The listing builds one solid part. Answer for the finished solid, in the listing's coordinates (mm). Face numbers are marked on the shaded views. A direction names the side the tool comes from. Coordinates: 2 decimals unless noted, no trailing zeros. Order: outer loops, then holes, each group sorted by start corner. A loop starts at its lowest first (then second) coordinate and runs counter-clockwise, first axis right, second up.
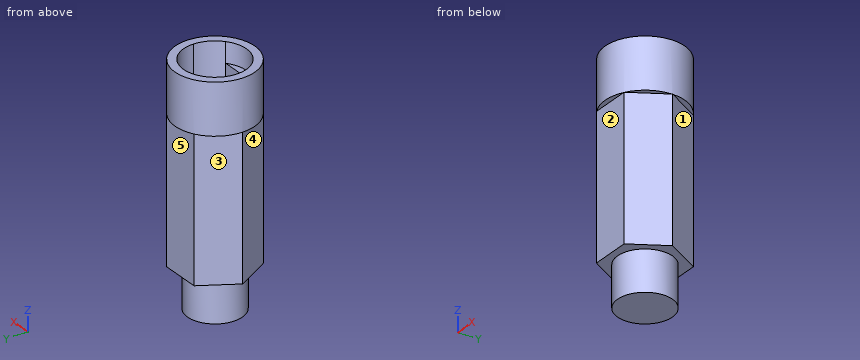
```python
from build123d import *

# Parameters (mm, degrees)
BOSS_EXTRUDE1_DEPTH = 14
SKETCH2_R           = 3.925
BOSS_EXTRUDE2_DEPTH = 5
SKETCH3_R           = 2.7
BOSS_EXTRUDE3_DEPTH = 4
CUT_EXTRUDE1_DEPTH  = 16
SKETCH5_R           = 3.1
CUT_EXTRUDE2_DEPTH  = 2


with BuildPart() as part:
    # Sketch1 → Boss-Extrude1 (new body)
    with BuildSketch(Plane.XY):
        Polygon((3.95, 0), (1.975, 3.420800345), (-1.975, 3.420800345), (-3.95, 0), (-1.975, -3.420800345), (1.975, -3.420800345), align=None)
    extrude(amount=BOSS_EXTRUDE1_DEPTH)

    # Sketch2 → Boss-Extrude2 (add)
    with BuildSketch(Plane.XY.offset(14)):
        with Locations(Location((0, 0, 0), (0, 0, 180.63826759))):
            Circle(SKETCH2_R)
    extrude(amount=BOSS_EXTRUDE2_DEPTH)

    # Sketch3 → Boss-Extrude3 (add)
    with BuildSketch(Plane(origin=(0, 0, 0), x_dir=(-1, 0, 0), z_dir=(0, 0, -1))):
        Circle(SKETCH3_R)
    extrude(amount=BOSS_EXTRUDE3_DEPTH)

    # Sketch4 → Cut-Extrude1 (cut)
    with BuildSketch(Plane.XY.offset(19)):
        with BuildLine():
            ThreePointArc((3.1, 0), (-1.328036289, 2.801128275), (-1.962141687, -2.4))
            Line((-1.962141687, -2.4), (1.962141687, -2.4))
            ThreePointArc((1.962141687, -2.4), (2.801128275, -1.328036289), (3.1, 0))
        make_face()
    extrude(amount=-CUT_EXTRUDE1_DEPTH, mode=Mode.SUBTRACT)

    # Sketch5 → Cut-Extrude2 (cut)
    with BuildSketch(Plane.XY.offset(19)):
        Circle(SKETCH5_R)
    extrude(amount=-CUT_EXTRUDE2_DEPTH, mode=Mode.SUBTRACT)


solid = part.part
```
1) A cutting plane is placed at C-C, the plane y = 0.5. Write down the section's boundary in (x, z), plus the area to 3 significant figures.
2) Straight lines are drawn through the part: probe 1 along Y at (x, z) = (0, 14.5) (3 decimals); probe 2 along X at (y, z) = (0, 17) (3 decimals); probe 3 along Y at (x, z) = (0, 10). For each, find the intervals that lie inside material, in ascending order.
3) A cutting plane is placed at A-A, the plane z = 11.5. Write down the section's boundary in (x, y) (3 decimals), plus the area to 3 significant figures.
4) For the marked faces 1, 2, 3, 4 and 5, determine the directions among +Z, -Z, +X, -X, +Y, -Y from which every point of the face is accessible in a straight line to the end or side of a thin tool.
5) A cutting plane is placed at B-B, the plane x = 0. Write down the section's boundary in (y, z) (3 decimals).
6) A cutting plane is placed at D-D, the plane z = -2. Write down the section's boundary in (x, y), plus the area to 3 significant figures.
7) Each of these flat-tipped pins is pushed along its axis until it touches: P1, Ø1.5, axis at y = -1.5, z = 0, coming from the +X side; P2, Ø2, axis at x = -1.5, z = 7, coming from the -Y side; P3, Ø0.6, axis at x = 3, y = -2, coming from the -Z side. Where does it stop, or does it pass through?
Working result:
1. outline: (-3.89, 14) - (-3.66, 14) - (-3.66, 0) - (-2.65, 0) - (-2.65, -4) - (2.65, -4) - (2.65, 0) - (3.66, 0) - (3.66, 14) - (3.89, 14) - (3.89, 19) - (3.06, 19) - (3.06, 3) - (-3.06, 3) - (-3.06, 19) - (-3.89, 19) - close
1. area: 64.8 mm2
2. probe 1: y = -3.925 to -2.4, 3.1 to 3.925
2. probe 2: x = -3.925 to -3.1, 3.1 to 3.925
2. probe 3: y = -3.42 to -2.4, 3.1 to 3.42
3. outline: (-3.95, 0) - (-1.975, -3.421) - (1.975, -3.421) - (3.95, 0) - (1.975, 3.421) - (-1.975, 3.421) - close; hole (-1.962, -2.4) - (1.962, -2.4) arc R3.1 ccw (long way) to start
3. area: 12.2 mm2
4. face 1: -Z, +X, +Y
4. face 2: -Z, +X, -X, -Y
4. face 3: -Z, -X, +Y
4. face 4: -Z, -X, -Y
4. face 5: -Z, +X, -X, +Y
5. outline: (-3.925, 14) - (-3.421, 14) - (-3.421, 0) - (-2.7, 0) - (-2.7, -4) - (2.7, -4) - (2.7, 0) - (3.421, 0) - (3.421, 14) - (3.925, 14) - (3.925, 19) - (3.1, 19) - (3.1, 3) - (-2.4, 3) - (-2.4, 17) - (-3.1, 17) - (-3.1, 19) - (-3.925, 19) - close
6. outline: circle Ø5.4 at (0, 0)
6. area: 22.9 mm2
7. P1: stops at x = 3.52
7. P2: stops at y = -3.42
7. P3: stops at z = 0
